```python
from build123d import *

# Parameters (mm, degrees)
SKETCH1_R               = 3.9
BOSS_EXTRUDE1_DEPTH     = 7
SKETCH2_R               = 4.7
BOSS_EXTRUDE2_DEPTH     = 2.5
CHAMFER1_SIZE           = 0.8
SKETCH3_R               = 3.4
SKETCH3_R_2             = 2.4
BOSS_EXTRUDE3_DEPTH     = 5.6
SKETCH4_R               = 2.05
BOSS_EXTRUDE4_DEPTH     = 9.1
SKETCH5_R               = 2.8
BOSS_EXTRUDE5_DEPTH     = 3
FILLET1_SIZE            = 0.5
FILLET1_SIZE_2          = 2.75
SKETCH6_W               = 0.5
SKETCH6_H               = 2.9
BOSS_EXTRUDE6_DEPTH     = 6.2
CUT_EXTRUDE1_DEPTH      = 6.2
CUT_EXTRUDE1_DEPTH_BACK = 6.2
SKETCH7_R               = 0.5


# Some blends are built 0.0001 mm under size
with BuildPart() as part:
    # Sketch1 → Boss-Extrude1 (new body)
    with BuildSketch(Plane(origin=(0, 0, 0), x_dir=(1, 0, 0), z_dir=(0, 1, 0))):
        with Locations(Location((0, 0, 0), (0, 0, 270))):
            Circle(SKETCH1_R)
    extrude(amount=-BOSS_EXTRUDE1_DEPTH)

    # Sketch2 → Boss-Extrude2 (add)
    with BuildSketch(Plane(origin=(0, 0, 0), x_dir=(1, 0, 0), z_dir=(0, 1, 0))):
        with Locations(Location((0, 0, 0), (0, 0, 270))):
            Circle(SKETCH2_R)
    extrude(amount=BOSS_EXTRUDE2_DEPTH)

    # Chamfer1
    chamfer1_edges = [part.edges().sort_by_distance(p)[0] for p in [
        (0, 0, -4.7),
    ]]
    chamfer(chamfer1_edges, length=CHAMFER1_SIZE - 0.0001)  # a hair under: the kernel refuses the full size

    # Sketch3 → Boss-Extrude3 (add)
    with BuildSketch(Plane(origin=(0, 2.5, 0), x_dir=(1, 0, 0), z_dir=(0, 1, 0))):
        with Locations(Location((0, 0, 0), (0, 0, 270))):
            Circle(SKETCH3_R)
        with Locations(Location((0, 0, 0), (0, 0, 270))):
            Circle(SKETCH3_R_2, mode=Mode.SUBTRACT)
    extrude(amount=BOSS_EXTRUDE3_DEPTH)

    # Sketch4 → Boss-Extrude4 (add)
    with BuildSketch(Plane(origin=(0, 2.5, 0), x_dir=(1, 0, 0), z_dir=(0, 1, 0))):
        with Locations(Location((0, 0, 0), (0, 0, 270))):
            Circle(SKETCH4_R)
    extrude(amount=BOSS_EXTRUDE4_DEPTH)

    # Sketch5 → Boss-Extrude5 (add)
    with BuildSketch(Plane(origin=(0, 11.6, 0), x_dir=(1, 0, 0), z_dir=(0, 1, 0))):
        with Locations(Location((0, 0, 0), (0, 0, 270))):
            Circle(SKETCH5_R)
    extrude(amount=BOSS_EXTRUDE5_DEPTH)

    # Fillet1
    # an asymmetric fillet: 2.75, 0.5 mm, written as the material it takes off along each edge
    with BuildSketch(Plane(origin=(0, 14.6, 0), x_dir=(0, 0, 1), z_dir=(-1, 0, 0))) as fillet1_piece_1:
        with BuildLine():
            Bezier((2.8, -FILLET1_SIZE), (2.8, 0), (2.8 - FILLET1_SIZE_2, 0), weights=[1, 0.707106781, 1])
            Line((2.8 - FILLET1_SIZE_2, 0), (2.8, 0))
            Line((2.8, 0), (2.8, -FILLET1_SIZE))
        make_face()
    revolve(axis=Axis((0, 14.6, 0), (0, 1, 0)), mode=Mode.SUBTRACT)

    # Sketch6 → Boss-Extrude6 (add)
    with BuildSketch(Plane.XZ.offset(7)):
        with Locations((-2.4, 0)):
            Rectangle(SKETCH6_W, SKETCH6_H)
        with Locations((2.4, 0)):
            Rectangle(SKETCH6_W, SKETCH6_H)
    extrude(amount=BOSS_EXTRUDE6_DEPTH)

    # Sketch7 → Cut-Extrude1 (cut, two sides: drawn at the far end of the back side and taken through both)
    with BuildSketch(Plane(origin=(0, 0, 0), x_dir=(0, 0, -1), z_dir=(1, 0, 0)).offset(-CUT_EXTRUDE1_DEPTH_BACK)):
        with BuildLine():
            ThreePointArc((-1.206978138, -10.946443049), (-0.891390932, -9.679801587), (-1.45, -8.5))
            Line((-1.45, -8.5), (-1.45, -11.75))
            ThreePointArc((-1.45, -11.75), (-1.387915397, -11.330249062), (-1.206978138, -10.946443049))
        make_face()
        with BuildLine():
            ThreePointArc((1.45, -11.749999997), (1.025304834, -12.775304832), (0, -13.2))
            Line((0, -13.2), (1.45, -13.2))
            Line((1.45, -13.2), (1.45, -11.749999997))
        make_face()
        with BuildLine():
            ThreePointArc((0, -13.2), (-1.025304833, -12.775304833), (-1.45, -11.75))
            Line((-1.45, -11.75), (-1.45, -13.2))
            Line((-1.45, -13.2), (0, -13.2))
        make_face()
        with BuildLine():
            ThreePointArc((1.206978138, -10.946443049), (1.387915397, -11.330249061), (1.45, -11.749999997))
            Line((1.45, -11.749999997), (1.45, -8.5))
            ThreePointArc((1.45, -8.5), (0.891390932, -9.679801587), (1.206978138, -10.946443049))
        make_face()
        with Locations(Location((0, -11.75, 0), (0, 0, 180))):
            Circle(SKETCH7_R)
    extrude(amount=CUT_EXTRUDE1_DEPTH + CUT_EXTRUDE1_DEPTH_BACK, mode=Mode.SUBTRACT)


solid = part.part
```
Can you work these out from the model? Positions are in its coordinate system, mm. A direction names the side the tool comes from. Round coordinates to 2 decimals unless told otherwise and drop trailing zeros. Loops run counter-clockwise (first coordinate to the right, second up) from the corner with the lowest first, then second, coordinate; pieces in that order, holes last. Notation, with made-up numbers: (89.25, -3.75) -> (147.25, -3.75) arc R24 ccw to (147.25, 8.25) -> close; hole circle Ø5 at (41.5, 83.25). An arc over 180 degrees is marked (long way). Answer in a Markdown table with one row per item.
Item 1: We'd pull the mould along Z, two halves only. Please class faces 1 (the cylindrical face through (1.412, 1.638, 4.483)), 2 (the cylindrical face through (2.396, -11.306, 0.231)), 3 (the cylindrical face through (2.033, 6.986, -0.267)), 4 (the flat face through (-2.15, -10, 0)): released by +Z, released by -Z, zero draft, split by the parting line, or undercut.
Answer block:
| item | result |
|---|---|
| face 1 | split by the parting line |
| face 2 | undercut |
| face 3 | undercut |
| face 4 | zero draft |
Item 2: On a 3-axis mill with a long thin cutter (end or side, diameter ignored), from which of +Z, -Z, +X, -X, +Y, -Y can I reach the whole of each face in a straight line? I mean faces 5 (the cylindrical face through (-3.32, 5.26, -0.74)), 6 (the flat face through (-2.2, 8.1, 1.5)), 7 (the flat face through (2.15, -10, 0)). Say none if no direction works.
Answer block:
| item | result |
|---|---|
| face 5 | +Y |
| face 6 | none |
| face 7 | +Z, -Z, -Y |
Item 3: Suppose I cut it at C-C, the plane y = 2. List the corners of the cut face in (x, z) for me, plus the area to 3 significant figures.
Answer block:
| item | result |
|---|---|
| outline | circle Ø9.4 at (0, 0) |
| area | 69.4 mm² |
Item 4: If I drill on probe 1 along X at (y, z) = (6.7, 0); probe 2 along Z at (x, y) = (-1.25, 8); probe 3 along Y at (x, z) = (3.25, 1.5), over which ranges is the centre line in solid material (lowest first)?
Answer block:
| item | result |
|---|---|
| probe 1 | -3.4 to -2.4, -2.05 to 2.05, 2.4 to 3.4 |
| probe 2 | -3.16 to -2.05, -1.62 to 1.62, 2.05 to 3.16 |
| probe 3 | -7 to 2.5 |
Item 5: Suppose I cut it at A-A, the plane y = -7.75. List the corners of the cut face in (x, z) for me, plus the area to 3 significant figures.
Answer block:
| item | result |
|---|---|
| outline | (-2.65, -1.45) -> (-2.15, -1.45) -> (-2.15, 1.45) -> (-2.65, 1.45) -> close; (2.15, -1.45) -> (2.65, -1.45) -> (2.65, 1.45) -> (2.15, 1.45) -> close |
| area | 2.90 mm² |
Item 6: Suppose I cut it at B-B, the plane y = 7.5. List the corners of the cut face in (x, z) for me.
Answer block:
| item | result |
|---|---|
| outline | circle Ø6.8 at (0, 0); circle Ø4.1 at (0, 0); hole circle Ø4.8 at (0, 0) |
Item 7: Will these pins go through, and if not, where does the flat tip stop? P1, Ø3, axis at y = -10.5, z = 0, coming from the -X side; P2, Ø2.5, axis at y = -9.5, z = 0.5, coming from the +X side; P3, Ø2, axis at x = 2.5, z = -3, coming from the -Y side.
Answer block:
| item | result |
|---|---|
| P1 | x = -2.65 |
| P2 | x = 2.65 |
| P3 | y = -7 |
